from build123d import *

# Parameters (mm, degrees)
SKETCH1_W           = 54.9
SKETCH1_H           = 8
SKETCH1_R           = 2.97
BOSS_EXTRUDE1_DEPTH = 1.12
SKETCH2_W           = 56.9
SKETCH2_H           = 10
SKETCH2_R           = 2.97
BOSS_EXTRUDE3_DEPTH = 2.5


with BuildPart() as part:
    # Sketch1 → Boss-Extrude1 (new body)
    with BuildSketch(Plane.XY):
        with Locations((-189.35, 6)):
            Rectangle(SKETCH1_W, SKETCH1_H)
        with Locations((-165.9, 6)):
            Circle(SKETCH1_R, mode=Mode.SUBTRACT)
        with Locations((-213.3, 6)):
            Circle(SKETCH1_R, mode=Mode.SUBTRACT)
    extrude(amount=BOSS_EXTRUDE1_DEPTH)

    # Sketch2 → Boss-Extrude3 (add)
    with BuildSketch(Plane.XY.offset(1.12)):
        with Locations((-189.35, 6)):
            Rectangle(SKETCH2_W, SKETCH2_H)
        with Locations((-213.3, 6)):
            Circle(SKETCH2_R, mode=Mode.SUBTRACT)
        with Locations((-165.9, 6)):
            Circle(SKETCH2_R, mode=Mode.SUBTRACT)
    extrude(amount=BOSS_EXTRUDE3_DEPTH)


solid = part.part
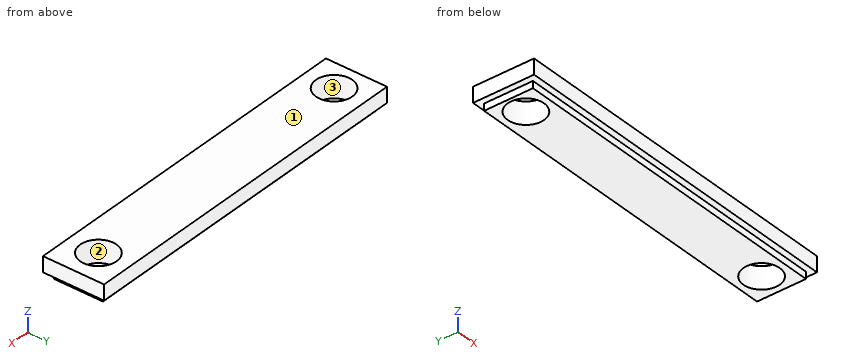
Work out the finished part from the listing and answer in its coordinate system (mm). Face numbers are marked on the shaded views. Round coordinates to 2 decimals unless told otherwise and drop trailing zeros. Write each loop counter-clockwise with the first axis right and the second up, starting at its lowest first coordinate (ties: lowest second). Pieces come first, ordered by that corner, then holes. Notation, with made-up numbers: (-11, -8) -> (-2, -8) arc R30 ccw to (-2, 24) -> close; hole circle Ø10 at (80.5, -38). An arc over 180 degrees is marked (long way). Answer as CSV lines item,"result". Start each with the question number.
(1) The part is cut by section C-C, the plane z = 2.3. Give the vertices of the cut face in (x, y), then the cut area to 3 significant figures.
(2) The part is cut by section A-A, the plane y = 6. Give the vertices of the cut face in (x, z).
(3) The mould has two halves that part along Y. Classify the marked faces 1, 2 and 3: +Y half, -Y half, draft (parallel to the pull), parting line (faces both ways), or undercut.
(4) The part is cut by section B-B, the plane x = -165.9. Give the vertices of the cut face in (y, z), then the cut area to 3 significant figures.
(5) Find the intervals of material crossed by probe 1 along Y at (x, z) = (-165.9, 1.8); probe 2 along X at (y, z) = (3.5, 0.5); probe 3 along Z at (x, y) = (-190, 10.25), in increasing order.
(6) Each of these flat-tipped pins is pushed along its axis until it touches: pin 1 (5 mm diameter, centred on x = -165.9, y = 6, fed in from -Z); pin 2 (0.9 mm diameter, centred on x = -201, z = 0.5, fed in from -Y). Where does it stop, or does it pass through?
(7) The part is cut by section D-D, the plane x = -200. Give the vertices of the cut face in (y, z), then the cut area to 3 significant figures.
Output values:
1,outline,"(-217.8, 1) -> (-160.9, 1) -> (-160.9, 11) -> (-217.8, 11) -> close; hole circle Ø5.94 at (-213.3, 6); hole circle Ø5.94 at (-165.9, 6)"
1,area,"514 mm²"
2,outline,"(-217.8, 1.12) -> (-216.8, 1.12) -> (-216.8, 0) -> (-216.27, 0) -> (-216.27, 3.62) -> (-217.8, 3.62) -> close; (-210.33, 0) -> (-168.87, 0) -> (-168.87, 3.62) -> (-210.33, 3.62) -> close; (-162.93, 0) -> (-161.9, 0) -> (-161.9, 1.12) -> (-160.9, 1.12) -> (-160.9, 3.62) -> (-162.93, 3.62) -> close"
3,face 1,"draft"
3,face 2,"undercut"
3,face 3,"undercut"
4,outline,"(1, 1.12) -> (2, 1.12) -> (2, 0) -> (3.03, 0) -> (3.03, 3.62) -> (1, 3.62) -> close; (8.97, 0) -> (10, 0) -> (10, 1.12) -> (11, 1.12) -> (11, 3.62) -> (8.97, 3.62) -> close"
4,area,"12.5 mm²"
5,probe 1,"y = 1 to 3.03, 8.97 to 11"
5,probe 2,"x = -216.8 to -214.9, -211.7 to -167.5, -164.3 to -161.9"
5,probe 3,"z = 1.12 to 3.62"
6,pin 1,"passes through"
6,pin 2,"stops at y = 2"
7,outline,"(1, 1.12) -> (2, 1.12) -> (2, 0) -> (10, 0) -> (10, 1.12) -> (11, 1.12) -> (11, 3.62) -> (1, 3.62) -> close"
7,area,"34.0 mm²"
